Source: three-view drawing plus pictorial views. Frame: mm from the lowest corner of the part. A direction names the side the tool comes from. Give positions to 0.01 mm unless a question says otherwise; leave off trailing zeros. Loops run counter-clockwise (first coordinate to the right, second up) from the corner with the lowest first, then second, coordinate; pieces in that order, holes last. Notation, with made-up numbers: M 54,-19.75 L 72,-19.75 A21 cw 72,10.25 Z; hole C 51,-20.5 d8. An arc over 180 degrees is marked long. Put each result on its own line as item: value. Start each with the question number.
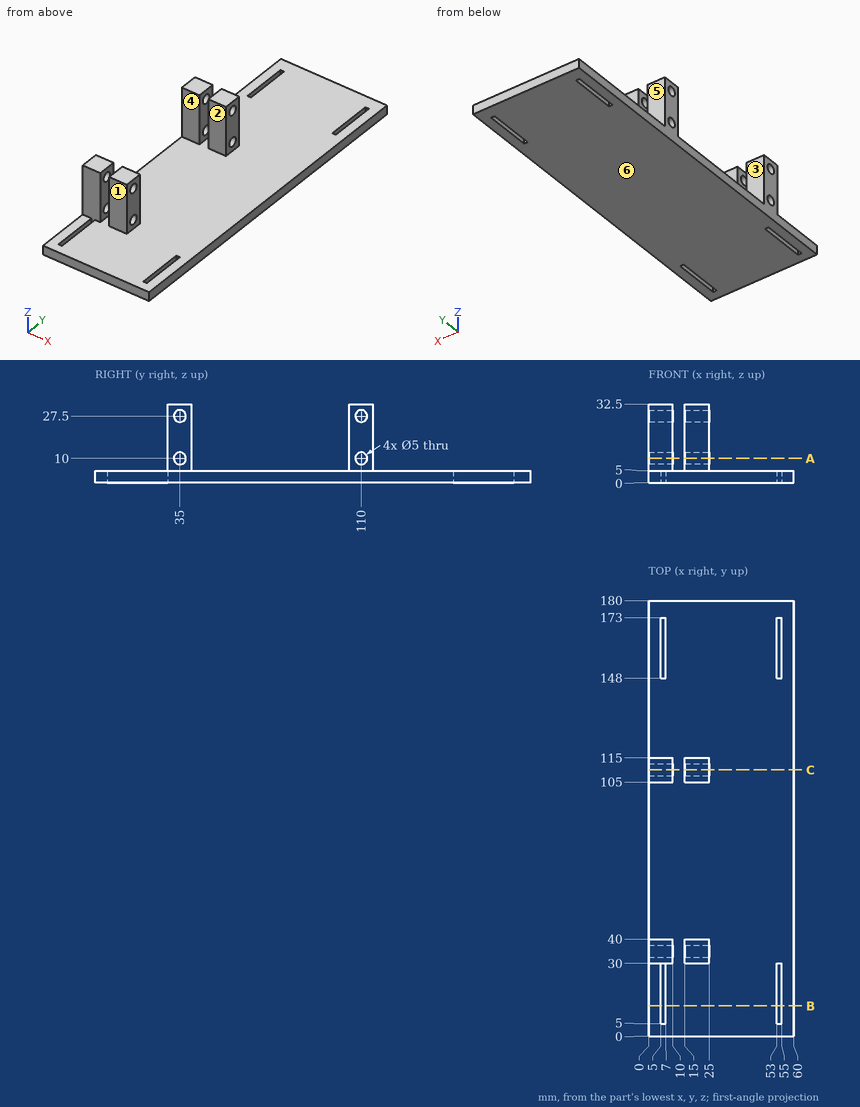
1. Section B-B, the plane y = 12.5. Output: boundary loops of the cut face in (x, z), plus the area to 3 significant figures.
2. Ray query, line 1 (Y direction, x = 18.5, z = 27.5); line 2 (X direction, y = 114, z = 24); line 3 (Y direction, x = 3, z = 14). Return the intervals inside material, ascending.
3. Pull-direction query (Y, two-part tool) for the marked faces 3, 4, 5 and 6; classes: released by +Y, released by -Y, zero draft, split by the parting line, or undercut.
4. Section C-C, the plane y = 110. Output: boundary loops of the cut face in (x, z), plus the area to 3 significant figures.
5. Contact query for flat-ended pins moving along their axis: pin 1 (3 mm diameter, centred on y = 109.5, z = 22, fed in from +X); pin 2 (6 mm diameter, centred on x = 14, z = 21, fed in from +Y); pin 3 (8 mm diameter, centred on x = 18.5, z = 18, fed in from -Y). Output: stop coordinate, or through.
6. Section A-A, the plane z = 10. State how many separate pieces and enclosed holes the cut face has, plus the area to 3 significant figures.
7. Set-up query: the marked faces 1 and 2. Return all of +Z, -Z, +X, -X, +Y, -Y with unobstructed straight access to the full face (end or side cutting, diameter ignored); none if empty.
Results found:
1. outline: M 0,0 L 5,0 L 5,5 L 0,5 Z; M 7,0 L 53,0 L 53,5 L 7,5 Z; M 55,0 L 60,0 L 60,5 L 55,5 Z
1. area: 280 mm²
2. line 1: 30 to 32.5, 37.5 to 40, 105 to 107.5, 112.5 to 115
2. line 2: 0 to 10, 15 to 25
2. line 3: 30 to 40, 105 to 115
3. face 3: undercut
3. face 4: undercut
3. face 5: released by +Y
3. face 6: zero draft
4. outline: M 0,0 L 60,0 L 60,5 L 25,5 L 25,7.5 L 15,7.5 L 15,5 L 10,5 L 10,7.5 L 0,7.5 Z; M 0,12.5 L 10,12.5 L 10,25 L 0,25 Z; M 0,30 L 10,30 L 10,32.5 L 0,32.5 Z; M 15,12.5 L 25,12.5 L 25,25 L 15,25 Z; M 15,30 L 25,30 L 25,32.5 L 15,32.5 Z
4. area: 650 mm²
5. pin 1: x = 25
5. pin 2: y = 115
5. pin 3: y = 30
6. separate pieces: 8
6. enclosed holes: 0
6. area: 200 mm²
7. face 1: +Z, +X, -X, -Y
7. face 2: +Z, +X, -X
